The listing builds one solid part. Answer for the finished solid, in the listing's coordinates (mm). A direction names the side the tool comes from. Round coordinates to 2 decimals unless told otherwise and drop trailing zeros. Write each loop counter-clockwise with the first axis right and the second up, starting at its lowest first coordinate (ties: lowest second). Pieces come first, ordered by that corner, then holes. Notation, with made-up numbers: (-35, 72.5) - (-4, 72.5) arc R33 cw to (-4, 101.5) - close; hole circle Ø3 at (57, 7). An arc over 180 degrees is marked (long way). Answer in a Markdown table with one row per item.
from build123d import *

# Parameters (mm, degrees)
ESQUISSE1_W        = 80
ESQUISSE1_H        = 100
BOSS_EXTRU_1_DEPTH = 5
ESQUISSE3_W        = 5
ESQUISSE3_H        = 100
BOSS_EXTRU_2_DEPTH = 20
ESQUISSE4_W        = 5
ESQUISSE4_H        = 100
BOSS_EXTRU_3_DEPTH = 12


with BuildPart() as part:
    # Esquisse1 → Boss.-Extru.1 (new body)
    with BuildSketch(Plane(origin=(0, 0, 0), x_dir=(1, 0, 0), z_dir=(0, 1, 0))):
        Rectangle(ESQUISSE1_W, ESQUISSE1_H)
    extrude(amount=BOSS_EXTRU_1_DEPTH)

    # Esquisse3 → Boss.-Extru.2 (add)
    with BuildSketch(Plane.XZ):
        with Locations((-37.5, 0)):
            Rectangle(ESQUISSE3_W, ESQUISSE3_H)
        with Locations((-30.5, 0)):
            Rectangle(ESQUISSE3_W, ESQUISSE3_H)
        with Locations((30.5, 0)):
            Rectangle(ESQUISSE3_W, ESQUISSE3_H)
        with Locations((37.5, 0)):
            Rectangle(ESQUISSE3_W, ESQUISSE3_H)
    extrude(amount=BOSS_EXTRU_2_DEPTH)

    # Esquisse4 → Boss.-Extru.3 (add)
    with BuildSketch(Plane(origin=(0, 5, 0), x_dir=(1, 0, 0), z_dir=(0, 1, 0))):
        with Locations((-12.5, 0)):
            Rectangle(ESQUISSE4_W, ESQUISSE4_H)
        with Locations((12.5, 0)):
            Rectangle(ESQUISSE4_W, ESQUISSE4_H)
    extrude(amount=BOSS_EXTRU_3_DEPTH)


solid = part.part
(1) Flat-ended cylindrical pins translate along their axes: pin 1 (1.5 mm diameter, centred on y = 13, z = -8, fed in from +X); pin 2 (8 mm diameter, centred on x = -3, z = -10.5, fed in from -Y); pin 3 (12.5 mm diameter, centred on x = -21.5, z = 9.5, fed in from +Y). Find the tip coordinate at first contact, or state that the pin passes through.
Checked values:
| item | result |
|---|---|
| pin 1 | stops at x = 15 |
| pin 2 | stops at y = 0 |
| pin 3 | stops at y = 5 |
(2) Section C-C (y = 6.5) is taken. Give the vertices of the cut face in (x, z), and give its area (3 significant figures).
Checked values:
| item | result |
|---|---|
| outline | (-15, -50) - (-10, -50) - (-10, 50) - (-15, 50) - close; (10, -50) - (15, -50) - (15, 50) - (10, 50) - close |
| area | 1,000 mm2 |
(3) Section B-B (z = 34) is taken. Give the vertices of the cut face in (x, y), and give its area (3 significant figures).
Checked values:
| item | result |
|---|---|
| outline | (-40, -20) - (-35, -20) - (-35, 0) - (-33, 0) - (-33, -20) - (-28, -20) - (-28, 0) - (28, 0) - (28, -20) - (33, -20) - (33, 0) - (35, 0) - (35, -20) - (40, -20) - (40, 5) - (15, 5) - (15, 17) - (10, 17) - (10, 5) - (-10, 5) - (-10, 17) - (-15, 17) - (-15, 5) - (-40, 5) - close |
| area | 920 mm2 |
(4) For faces 4 (the flat face through (0, 5, -1)), 5 (the flat face through (27, 5, -1)), 6 (the flat face through (0, 0, -1)), 7 (the flat face through (-15, 11, 1)), determine the directions among +Z, -Z, +X, -X, +Y, -Y from which every point of the face is accessible in a straight line to the end or side of a thin tool.
Checked values:
| item | result |
|---|---|
| face 4 | +Z, -Z, +Y |
| face 5 | +Z, -Z, +X, +Y |
| face 6 | +Z, -Z, -Y |
| face 7 | +Z, -Z, -X, +Y |
(5) For a pull along X with two mould halves and no side action, classify faces 1 (the flat face through (40, -8, 1)), 2 (the flat face through (-13, 17, -1)), 3 (the flat face through (-28, -10, -1)) as pulls with the +X half, pulls with the -X half, needs draft (parallel to the pull), parting line crosses it, or undercut.
Checked values:
| item | result |
|---|---|
| face 1 | pulls with the +X half |
| face 2 | needs draft |
| face 3 | undercut |
(6) Section D-D (x = -19) is taken. Give the vertices of the cut face in (y, z), and give its area (3 significant figures).
Checked values:
| item | result |
|---|---|
| outline | (0, -50) - (5, -50) - (5, 50) - (0, 50) - close |
| area | 500 mm2 |
(7) Section A-A (y = -17) is taken. Give the vertices of the cut face in (x, z), and give its area (3 significant figures).
Checked values:
| item | result |
|---|---|
| outline | (-40, -50) - (-35, -50) - (-35, 50) - (-40, 50) - close; (-33, -50) - (-28, -50) - (-28, 50) - (-33, 50) - close; (28, -50) - (33, -50) - (33, 50) - (28, 50) - close; (35, -50) - (40, -50) - (40, 50) - (35, 50) - close |
| area | 2,000 mm2 |
(8) Find the intervals of material crossed by line 1 (X direction, y = -6.5, z = -28.5); line 2 (X direction, y = 13.5, z = 28); line 3 (Y direction, x = -14, z = -28.5), in increasing order.
Checked values:
| item | result |
|---|---|
| line 1 | x = -40 to -35, -33 to -28, 28 to 33, 35 to 40 |
| line 2 | x = -15 to -10, 10 to 15 |
| line 3 | y = 0 to 17 |
